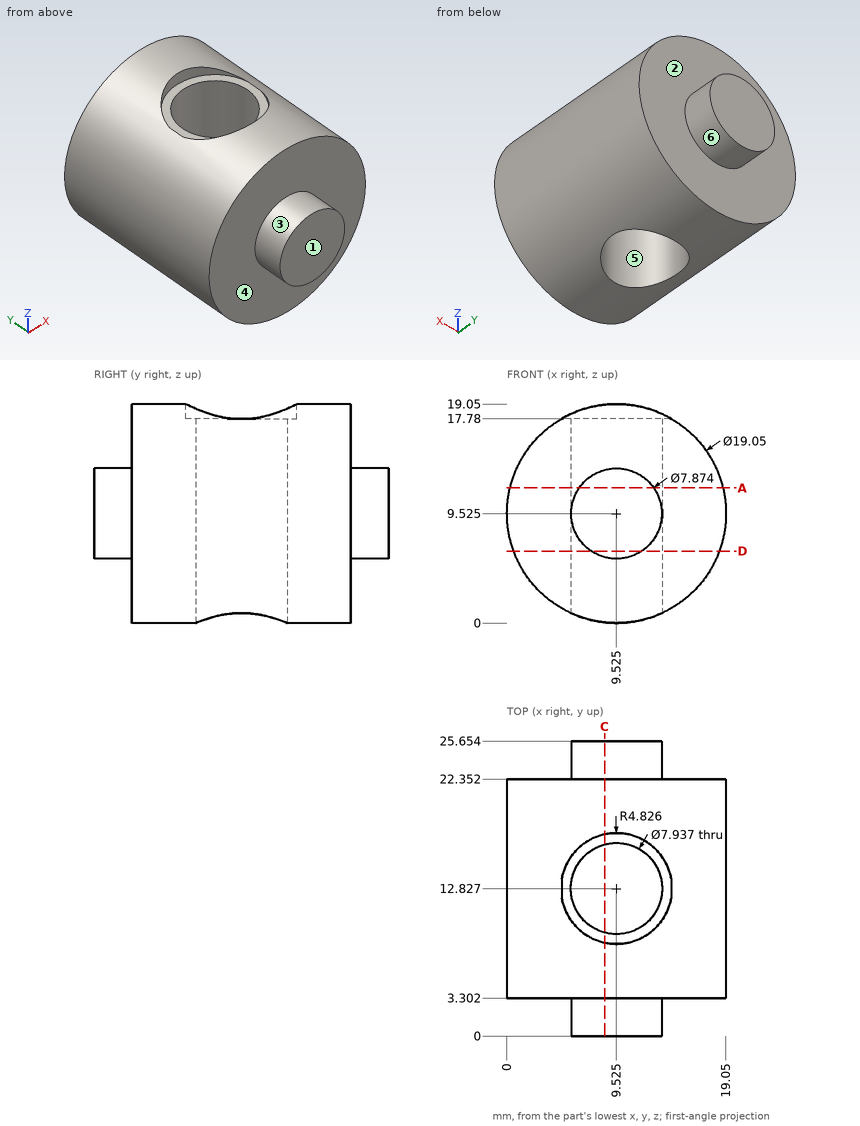
Study the drawing (mm; zero at the part's minimum x, y, z) and answer. A direction names the side the tool comes from. Coordinates: 2 decimals unless noted, no trailing zeros. Write each loop counter-clockwise with the first axis right and the second up, starting at its lowest first coordinate (ties: lowest second). Pieces come first, ordered by that corner, then holes. Notation, with made-up numbers: (-29, -14.5) - (22, -14.5) arc R32 ccw to (22, 16.5) - close; hole circle Ø6 at (-31.75, -14). An arc over 180 degrees is marked (long way). Return JSON: item names as keys, results as strings. Group by question number.
1. Which of the six approach directions +Z, -Z, +X, -X, +Y, -Y give full straight-line access (tool end or side, diameter ignored) to the marked faces 1, 2 and 3?
2. A cutting plane is placed at C-C, the plane x = 8.5. Determine the outline of the cut face in (y, z) (1 decimal).
3. A cutting plane is placed at D-D, the plane z = 6.25. Determine the outline of the cut face in (x, y) (1 decimal).
4. Determine the mould class of the marked faces 4, 5 and 6 for opening direction Y: released by +Y, released by -Y, zero draft, split by the parting line, or undercut.
5. A cutting plane is placed at A-A, the plane z = 11.75. Determine the outline of the cut face in (x, y) (1 decimal).
6. Given pin 1 (3 mm diameter, centred on x = 6, y = 9.5, fed in from -Z); pin 2 (4 mm diameter, centred on x = 5, y = 13.5, fed in from -Z); pin 3 (7.5 mm diameter, centred on x = 11.5, y = 12, fed in from +Z), each flat-ended and moving along its own axis, determine where each tip first touches the part or whether it passes through.
7. Straight lines are drawn through the part: L1, parallel to X at y = 11.5, z = 6.75 (1 decimal); L2, parallel to X at y = 10.75, z = 13.25 (1 decimal); L3, parallel to Y at x = 17, z = 4.75. For each, find the intervals that lie inside material, in ascending order.
Ans:
{
 "1": {"face 1": "+Z, -Z, +X, -X, -Y", "face 2": "+Y", "face 3": "-Y"},
 "2": {"outline": "(0, 5.7) - (3.3, 5.7) - (3.3, 0.1) - (9, 0.1) - (9, 17.8) - (8.1, 17.8) - (8.1, 19) - (3.3, 19) - (3.3, 13.3) - (0, 13.3) - close; (16.7, 0.1) - (22.4, 0.1) - (22.4, 5.7) - (25.7, 5.7) - (25.7, 13.3) - (22.4, 13.3) - (22.4, 19) - (17.5, 19) - (17.5, 17.8) - (16.7, 17.8) - close"},
 "3": {"outline": "(0.6, 3.3) - (7.3, 3.3) - (7.3, 0) - (11.7, 0) - (11.7, 3.3) - (18.5, 3.3) - (18.5, 22.4) - (11.7, 22.4) - (11.7, 25.7) - (7.3, 25.7) - (7.3, 22.4) - (0.6, 22.4) - close; hole circle Ø7.9 at (9.5, 12.8)"},
 "4": {"face 4": "released by -Y", "face 5": "undercut", "face 6": "zero draft"},
 "5": {"outline": "(0.3, 3.3) - (6.3, 3.3) - (6.3, 0) - (12.8, 0) - (12.8, 3.3) - (18.8, 3.3) - (18.8, 22.4) - (12.8, 22.4) - (12.8, 25.7) - (6.3, 25.7) - (6.3, 22.4) - (0.3, 22.4) - close; hole circle Ø7.9 at (9.5, 12.8)"},
 "6": {"pin 1": "z = 0.22", "pin 2": "z = 0.58", "pin 3": "z = 18.92"},
 "7": {"L1": "0.4 to 5.8, 13.3 to 18.6", "L2": "0.8 to 6.1, 12.9 to 18.3", "L3": "3.3 to 22.35"}
}
